from build123d import *

# Parameters (mm, degrees)
SKETCH1_R                                   = 107.5
SKETCH1_R_2                                 = 100
BOSS_EXTRUDE1_DEPTH                         = 187
BOSS_EXTRUDE2_DEPTH                         = 30
BOSS_EXTRUDE3_DEPTH                         = 20
FILLET1_R                                   = 30
FILLET2_R                                   = 10
SKETCH5_R                                   = 105
CUT_EXTRUDE1_DEPTH                          = 942
SKETCH6_R                                   = 107.5
BOSS_EXTRUDE6_DEPTH                         = 10
SKETCH7_R                                   = 107.5
SKETCH7_R_2                                 = 100
BOSS_EXTRUDE7_DEPTH                         = 200
SKETCH8_R                                   = 102.5
SKETCH8_R_2                                 = 95
BOSS_EXTRUDE8_DEPTH                         = 4
CUT_EXTRUDE2_START                          = -2.5
SKETCH9_R                                   = 102.5
CUT_EXTRUDE2_DEPTH                          = 2.5
SKETCH10_R                                  = 31
CUT_EXTRUDE3_DEPTH                          = 28
CBORE_FOR_M4_HEX_HEAD_CAP_SCREW1_AT_2_COUNT = 2
CBORE_FOR_M4_HEX_HEAD_CAP_SCREW1_AT_2_PITCH = 53.575680531
CBORE_FOR_M4_HEX_HEAD_CAP_SCREW1_AT_3_COUNT = 2
CBORE_FOR_M4_HEX_HEAD_CAP_SCREW1_AT_3_PITCH = 98.994949366
CBORE_FOR_M4_HEX_HEAD_CAP_SCREW1_AT_4_COUNT = 2
CBORE_FOR_M4_HEX_HEAD_CAP_SCREW1_AT_4_PITCH = 129.343134552
CBORE_FOR_M4_HEX_HEAD_CAP_SCREW1_AT_5_COUNT = 2
CBORE_FOR_M4_HEX_HEAD_CAP_SCREW1_AT_5_PITCH = 140
CBORE_FOR_M4_HEX_HEAD_CAP_SCREW1_AT_6_COUNT = 2
CBORE_FOR_M4_HEX_HEAD_CAP_SCREW1_AT_6_PITCH = 129.343134552
CBORE_FOR_M4_HEX_HEAD_CAP_SCREW1_AT_7_COUNT = 2
CBORE_FOR_M4_HEX_HEAD_CAP_SCREW1_AT_7_PITCH = 98.994949366
CBORE_FOR_M4_HEX_HEAD_CAP_SCREW1_AT_8_COUNT = 2
CBORE_FOR_M4_HEX_HEAD_CAP_SCREW1_AT_8_PITCH = 53.575680531
CBORE_FOR_M3_HEX_HEAD_CAP_SCREW1_AT_2_COUNT = 2
CBORE_FOR_M3_HEX_HEAD_CAP_SCREW1_AT_2_PITCH = 32.145408414
CBORE_FOR_M3_HEX_HEAD_CAP_SCREW1_AT_3_COUNT = 2
CBORE_FOR_M3_HEX_HEAD_CAP_SCREW1_AT_3_PITCH = 59.396969796
CBORE_FOR_M3_HEX_HEAD_CAP_SCREW1_AT_4_COUNT = 2
CBORE_FOR_M3_HEX_HEAD_CAP_SCREW1_AT_4_PITCH = 77.605880961
CBORE_FOR_M3_HEX_HEAD_CAP_SCREW1_AT_5_COUNT = 2
CBORE_FOR_M3_HEX_HEAD_CAP_SCREW1_AT_5_PITCH = 84.00000025
CBORE_FOR_M3_HEX_HEAD_CAP_SCREW1_AT_6_COUNT = 2
CBORE_FOR_M3_HEX_HEAD_CAP_SCREW1_AT_6_PITCH = 77.605880961
CBORE_FOR_M3_HEX_HEAD_CAP_SCREW1_AT_7_COUNT = 2
CBORE_FOR_M3_HEX_HEAD_CAP_SCREW1_AT_7_PITCH = 59.396969796
CBORE_FOR_M3_HEX_HEAD_CAP_SCREW1_AT_8_COUNT = 2
CBORE_FOR_M3_HEX_HEAD_CAP_SCREW1_AT_8_PITCH = 32.145408414
BOSS_EXTRUDE9_START                         = 237
SKETCH20_R                                  = 105
SKETCH20_R_2                                = 90
BOSS_EXTRUDE9_DEPTH                         = 237
SKETCH21_R                                  = 12
CUT_EXTRUDE4_DEPTH                          = 421


with BuildPart() as part:
    # Sketch1 → Boss-Extrude1 (new body)
    with BuildSketch(Plane.XY):
        Circle(SKETCH1_R)
        Circle(SKETCH1_R_2, mode=Mode.SUBTRACT)
    extrude(amount=BOSS_EXTRUDE1_DEPTH)

    # Sketch2 → Boss-Extrude2 (add)
    with BuildSketch(Plane(origin=(0, 0, 0), x_dir=(-1, 0, 0), z_dir=(0, 0, -1))):
        Polygon((-199.547059231, -71.978963263), (-71.978963263, 199.547059231), (63.784047984, 135.763011247), (199.547059231, 71.978963263), (71.978963263, -199.547059231), (-63.784047984, -135.763011247), align=None)
    extrude(amount=BOSS_EXTRUDE2_DEPTH)

    # Sketch3 → Boss-Extrude3 (add)
    with BuildSketch(Plane(origin=(0, 0, -30), x_dir=(-1, 0, 0), z_dir=(0, 0, -1))):
        Polygon((-199.547059231, -71.978963263), (71.978963263, -199.547059231), (199.547059231, 71.978963263), (-71.978963263, 199.547059231), align=None)
    extrude(amount=BOSS_EXTRUDE3_DEPTH)

    # Fillet1
    fillet1_edges = [part.edges().sort_by_distance(p)[0] for p in [
        (199.547059231, -71.978963263, -25),
        (-71.978963263, -199.547059231, -25),
        (-199.547059231, 71.978963263, -25),
        (71.978963263, 199.547059231, -25),
    ]]
    fillet(fillet1_edges, radius=FILLET1_R)

    # Fillet2
    fillet2_edges = [part.edges().sort_by_distance(p)[0] for p in [
        (-107.5, 0, 0),
    ]]
    fillet(fillet2_edges, radius=FILLET2_R)

    # Sketch5 → Cut-Extrude1 (cut)
    with BuildSketch(Plane(origin=(0, 0, -50), x_dir=(-1, 0, 0), z_dir=(0, 0, -1))):
        Circle(SKETCH5_R)
    extrude(amount=-CUT_EXTRUDE1_DEPTH, mode=Mode.SUBTRACT)

    # Sketch6 → Boss-Extrude6 (add)
    with BuildSketch(Plane.XY.offset(187)):
        with Locations(Location((0, 0, 0), (0, 0, 180))):
            Circle(SKETCH6_R)
    extrude(amount=BOSS_EXTRUDE6_DEPTH)

    # Sketch7 → Boss-Extrude7 (add)
    with BuildSketch(Plane.XY.offset(197)):
        with Locations(Location((0, 0, 0), (0, 0, 180))):
            Circle(SKETCH7_R)
        Circle(SKETCH7_R_2, mode=Mode.SUBTRACT)
    extrude(amount=BOSS_EXTRUDE7_DEPTH)

    # Sketch8 → Boss-Extrude8 (add)
    with BuildSketch(Plane.XY.offset(197)):
        Circle(SKETCH8_R)
        Circle(SKETCH8_R_2, mode=Mode.SUBTRACT)
    extrude(amount=BOSS_EXTRUDE8_DEPTH)

    # Sketch9 → Cut-Extrude2 (cut)
    with BuildSketch(Plane.XY.offset(397).offset(CUT_EXTRUDE2_START)):
        Circle(SKETCH9_R)
    extrude(amount=-CUT_EXTRUDE2_DEPTH, mode=Mode.SUBTRACT)

    # Sketch10 → Cut-Extrude3 (cut)
    with BuildSketch(Plane(origin=(0, 0, 187), x_dir=(-1, 0, 0), z_dir=(0, 0, -1))):
        Circle(SKETCH10_R)
    extrude(amount=-CUT_EXTRUDE3_DEPTH, mode=Mode.SUBTRACT)

    # Sketch13 → CBORE for M4 Hex Head Cap Screw1 (revolve, cut)
    with BuildSketch(Plane(origin=(23.75184564, 65.847170241, 197), x_dir=(0, -1, 0), z_dir=(1, 0, 0))):
        Polygon((0, 0), (0, 11.351936393), (2.25, 10), (2.25, 2.8), (5.5415, 2.8), (5.5415, 0.025), (5.5665, 0), align=None)
    cbore_for_m4_hex_head_cap_screw1 = revolve(axis=Axis((23.75184564, 65.847170241, 203.35), (0, 0, -1)), mode=Mode.SUBTRACT)

    # CBORE for M4 Hex Head Cap Screw1 at 2: CBORE for M4 Hex Head Cap Screw1 ×2
    with Locations(*[Vector(0.7392202149258387, -0.6734637880725266, 0) * (i * CBORE_FOR_M4_HEX_HEAD_CAP_SCREW1_AT_2_PITCH) for i in range(1, CBORE_FOR_M4_HEX_HEAD_CAP_SCREW1_AT_2_COUNT)]):
        add(cbore_for_m4_hex_head_cap_screw1, mode=Mode.SUBTRACT)

    # CBORE for M4 Hex Head Cap Screw1 at 3: CBORE for M4 Hex Head Cap Screw1 ×2
    with Locations(*[Vector(0.4252269925953868, -0.9050867388092054, 0) * (i * CBORE_FOR_M4_HEX_HEAD_CAP_SCREW1_AT_3_PITCH) for i in range(1, CBORE_FOR_M4_HEX_HEAD_CAP_SCREW1_AT_3_COUNT)]):
        add(cbore_for_m4_hex_head_cap_screw1, mode=Mode.SUBTRACT)

    # CBORE for M4 Hex Head Cap Screw1 at 4: CBORE for M4 Hex Head Cap Screw1 ×2
    with Locations(*[Vector(0.04649681533457415, -0.998918438193901, 0) * (i * CBORE_FOR_M4_HEX_HEAD_CAP_SCREW1_AT_4_PITCH) for i in range(1, CBORE_FOR_M4_HEX_HEAD_CAP_SCREW1_AT_4_COUNT)]):
        add(cbore_for_m4_hex_head_cap_screw1, mode=Mode.SUBTRACT)

    # CBORE for M4 Hex Head Cap Screw1 at 5: CBORE for M4 Hex Head Cap Screw1 ×2
    with Locations(*[Vector(-0.3393120805662469, -0.9406738605817666, 0) * (i * CBORE_FOR_M4_HEX_HEAD_CAP_SCREW1_AT_5_PITCH) for i in range(1, CBORE_FOR_M4_HEX_HEAD_CAP_SCREW1_AT_5_COUNT)]):
        add(cbore_for_m4_hex_head_cap_screw1, mode=Mode.SUBTRACT)

    # CBORE for M4 Hex Head Cap Screw1 at 6: CBORE for M4 Hex Head Cap Screw1 ×2
    with Locations(*[Vector(-0.6734637880725266, -0.7392202149258387, 0) * (i * CBORE_FOR_M4_HEX_HEAD_CAP_SCREW1_AT_6_PITCH) for i in range(1, CBORE_FOR_M4_HEX_HEAD_CAP_SCREW1_AT_6_COUNT)]):
        add(cbore_for_m4_hex_head_cap_screw1, mode=Mode.SUBTRACT)

    # CBORE for M4 Hex Head Cap Screw1 at 7: CBORE for M4 Hex Head Cap Screw1 ×2
    with Locations(*[Vector(-0.9050867388092054, -0.4252269925953869, 0) * (i * CBORE_FOR_M4_HEX_HEAD_CAP_SCREW1_AT_7_PITCH) for i in range(1, CBORE_FOR_M4_HEX_HEAD_CAP_SCREW1_AT_7_COUNT)]):
        add(cbore_for_m4_hex_head_cap_screw1, mode=Mode.SUBTRACT)

    # CBORE for M4 Hex Head Cap Screw1 at 8: CBORE for M4 Hex Head Cap Screw1 ×2
    with Locations(*[Vector(-0.9989184381939011, -0.046496815334574164, 0) * (i * CBORE_FOR_M4_HEX_HEAD_CAP_SCREW1_AT_8_PITCH) for i in range(1, CBORE_FOR_M4_HEX_HEAD_CAP_SCREW1_AT_8_COUNT)]):
        add(cbore_for_m4_hex_head_cap_screw1, mode=Mode.SUBTRACT)

    # Sketch19 → CBORE for M3 Hex Head Cap Screw1 (revolve, cut)
    with BuildSketch(Plane(origin=(14.251107426, 39.508302262, 197), x_dir=(0, -1, 0), z_dir=(1, 0, 0))):
        Polygon((0, 0), (0, 11.021463052), (1.7, 10), (1.7, 2), (4.6755, 2), (4.6755, 0.025), (4.7005, 0), align=None)
    cbore_for_m3_hex_head_cap_screw1 = revolve(axis=Axis((14.251107426, 39.508302262, 203.35), (0, 0, -1)), mode=Mode.SUBTRACT)

    # CBORE for M3 Hex Head Cap Screw1 at 2: CBORE for M3 Hex Head Cap Screw1 ×2
    with Locations(*[Vector(0.7392202149258387, -0.6734637880725266, 0) * (i * CBORE_FOR_M3_HEX_HEAD_CAP_SCREW1_AT_2_PITCH) for i in range(1, CBORE_FOR_M3_HEX_HEAD_CAP_SCREW1_AT_2_COUNT)]):
        add(cbore_for_m3_hex_head_cap_screw1, mode=Mode.SUBTRACT)

    # CBORE for M3 Hex Head Cap Screw1 at 3: CBORE for M3 Hex Head Cap Screw1 ×2
    with Locations(*[Vector(0.4252269925953868, -0.9050867388092055, 0) * (i * CBORE_FOR_M3_HEX_HEAD_CAP_SCREW1_AT_3_PITCH) for i in range(1, CBORE_FOR_M3_HEX_HEAD_CAP_SCREW1_AT_3_COUNT)]):
        add(cbore_for_m3_hex_head_cap_screw1, mode=Mode.SUBTRACT)

    # CBORE for M3 Hex Head Cap Screw1 at 4: CBORE for M3 Hex Head Cap Screw1 ×2
    with Locations(*[Vector(0.0464968153345742, -0.9989184381939011, 0) * (i * CBORE_FOR_M3_HEX_HEAD_CAP_SCREW1_AT_4_PITCH) for i in range(1, CBORE_FOR_M3_HEX_HEAD_CAP_SCREW1_AT_4_COUNT)]):
        add(cbore_for_m3_hex_head_cap_screw1, mode=Mode.SUBTRACT)

    # CBORE for M3 Hex Head Cap Screw1 at 5: CBORE for M3 Hex Head Cap Screw1 ×2
    with Locations(*[Vector(-0.3393120805662469, -0.9406738605817666, 0) * (i * CBORE_FOR_M3_HEX_HEAD_CAP_SCREW1_AT_5_PITCH) for i in range(1, CBORE_FOR_M3_HEX_HEAD_CAP_SCREW1_AT_5_COUNT)]):
        add(cbore_for_m3_hex_head_cap_screw1, mode=Mode.SUBTRACT)

    # CBORE for M3 Hex Head Cap Screw1 at 6: CBORE for M3 Hex Head Cap Screw1 ×2
    with Locations(*[Vector(-0.6734637880725266, -0.7392202149258387, 0) * (i * CBORE_FOR_M3_HEX_HEAD_CAP_SCREW1_AT_6_PITCH) for i in range(1, CBORE_FOR_M3_HEX_HEAD_CAP_SCREW1_AT_6_COUNT)]):
        add(cbore_for_m3_hex_head_cap_screw1, mode=Mode.SUBTRACT)

    # CBORE for M3 Hex Head Cap Screw1 at 7: CBORE for M3 Hex Head Cap Screw1 ×2
    with Locations(*[Vector(-0.9050867388092054, -0.4252269925953869, 0) * (i * CBORE_FOR_M3_HEX_HEAD_CAP_SCREW1_AT_7_PITCH) for i in range(1, CBORE_FOR_M3_HEX_HEAD_CAP_SCREW1_AT_7_COUNT)]):
        add(cbore_for_m3_hex_head_cap_screw1, mode=Mode.SUBTRACT)

    # CBORE for M3 Hex Head Cap Screw1 at 8: CBORE for M3 Hex Head Cap Screw1 ×2
    with Locations(*[Vector(-0.998918438193901, -0.046496815334574004, 0) * (i * CBORE_FOR_M3_HEX_HEAD_CAP_SCREW1_AT_8_PITCH) for i in range(1, CBORE_FOR_M3_HEX_HEAD_CAP_SCREW1_AT_8_COUNT)]):
        add(cbore_for_m3_hex_head_cap_screw1, mode=Mode.SUBTRACT)

    # Sketch20 → Boss-Extrude9 (add)
    with BuildSketch(Plane(origin=(0, 0, 187), x_dir=(-1, 0, 0), z_dir=(0, 0, -1)).offset(BOSS_EXTRUDE9_START)):
        Circle(SKETCH20_R)
        Circle(SKETCH20_R_2, mode=Mode.SUBTRACT)
    extrude(amount=-BOSS_EXTRUDE9_DEPTH)

    # Sketch21 → Cut-Extrude4 (cut)
    with BuildSketch(Plane.XY):
        with Locations((-159.637647385, 57.58317061)):
            Circle(SKETCH21_R)
        with Locations((57.58317061, 159.637647385)):
            Circle(SKETCH21_R)
        with Locations((159.637647385, -57.58317061)):
            Circle(SKETCH21_R)
        with Locations((-57.58317061, -159.637647385)):
            Circle(SKETCH21_R)
    extrude(amount=-CUT_EXTRUDE4_DEPTH, mode=Mode.SUBTRACT)


solid = part.part
Check sheet for the modelled part. Datum: model origin and axes. Units: mm. A direction names the side the tool comes from. Give positions to 0.01 mm unless a question says otherwise; leave off trailing zeros. Loops run counter-clockwise (first coordinate to the right, second up) from the corner with the lowest first, then second, coordinate; pieces in that order, holes last. Notation, with made-up numbers: M -33,68 L -29,68 A24 ccw -29,107 Z; hole C -26,45 d4. An arc over 180 degrees is marked long. Use a Markdown table: item, result. Add a question column.
Q1. Scan lines: line 1 along X through (y, z) = (-58.5, -27); line 2 along Z through (x, y) = (-107.5, -100.5); line 3 along Y through (x, z) = (29, 119.5). Record each from-to range of solid material in increasing order. Write a range as [from, to].
Q2. Tool access check on faces 4 (the cylindrical face through (95.38, 30.04, 295.16)), 5 (the cylindrical face through (-46.14, -156.03, -24.65)). Record the directions out of +Z, -Z, +X, -X, +Y, -Y that give a thin tool (end or side, any length) a straight path to the whole face; none if there is none.
Q3. Sectioned sample at A-A, the plane z = 368. Record the cut outline in (x, y).
Q4. Mould release check, pull along Z, two halves, no side actions. Record for faces 1 (the flat face through (-63, -27, 194.2)), 2 (the flat face through (98, -22, 392)), 3 (the cylindrical face through (-41.53, -79.845, 66.841)): pulls with the +Z half, pulls with the -Z half, needs draft (parallel to the pull), parting line crosses it, or undercut.
Q5. Sectioned sample at D-D, the plane z = 20. Record the cut outline in (x, y).
Q6. Go/stop test with flat-tipped pins: pin 1 (9 mm diameter, centred on x = 65.85, y = -23.75, fed in from +Z); pin 2 (11 mm diameter, centred on x = 17.86, y = -38.01, fed in from +Z); pin 3 (12 mm diameter, centred on x = -102.5, z = 28, fed in from -Y); pin 4 (19 mm diameter, centred on x = 57.58, y = 159.64, fed in from +Z). Record where each tip stops, or that it passes through.
Q7. Sectioned sample at C-C, the plane y = 128. Record the cut outline in (x, z), then the cut area to 3 significant figures.
Verdict:
| question | item | result |
|---|---|---|
| 1 | line 1 | [-138.25, -68.39], [68.39, 147.67], [171.6, 189.62] |
| 1 | line 2 | [-50, 0] |
| 1 | line 3 | [-103.51, -85.2], [85.2, 103.51] |
| 2 | face 4 | +Z |
| 2 | face 5 | +Z, -Z |
| 3 | outline | C 0,0 d215; hole C 0,0 d200 |
| 4 | face 1 | pulls with the +Z half |
| 4 | face 2 | undercut |
| 4 | face 3 | needs draft |
| 5 | outline | C 0,0 d215; hole C 0,0 d180 |
| 6 | pin 1 | z = 194.2 |
| 6 | pin 2 | z = 197 |
| 6 | pin 3 | y = -47.37 |
| 6 | pin 4 | through |
| 7 | outline | M -80.31,-50 L 105.59,-50 L 105.59,0 L -80.31,0 Z |
| 7 | area | 9,300 mm^2 |
